Here's how the part is built. I have some questions about the finished solid (model axes, mm). A direction names the side the tool comes from. Give positions to 0.01 mm unless a question says otherwise; leave off trailing zeros. Loops run counter-clockwise (first coordinate to the right, second up) from the corner with the lowest first, then second, coordinate; pieces in that order, holes last. Notation, with made-up numbers: (-26, -10) - (-11, -10) arc R30 ccw to (-11, 15) - close; hole circle Ø6 at (-24, -5). An arc over 180 degrees is marked (long way). Use a Markdown table: item, result.
from build123d import *

# Parameters (mm, degrees)
SM_BASE_FLANGE_1_DEPTH = 2.5
HOLE_WIZARD_M41_D      = 3.3
OTHER_START            = 45.056896686
OTHER_7_OUTLINE_R      = 1.65
OTHER_7_DEPTH          = 7.095461821
OTHER_START_2          = 22.961384977
OTHER_7_2_DEPTH        = 30
OTHER_START_3          = 31.461384977
OTHER_7_3_DEPTH        = 13
OTHER_START_4          = 39.611384977
OTHER_7_4_DEPTH        = 5.85
OTHER_START_5          = 30.461384977
OTHER_7_5_DEPTH        = 5.8499999
OTHER_7_6_DEPTH        = 8.5
OTHER_START_6          = 44.461384977
OTHER_7_7_DEPTH        = 8.5
OTHER_START_7          = 40.219785041
OTHER_7_8_DEPTH        = 2.5


with BuildPart() as part:
    # Базовая кромка1: sheet metal written as solids
    # Sketch 1 → Базовая кромка1 (new body)
    with BuildSketch(Plane.XY):
        Polygon((54.77467234, 44.461384977), (73.77467234, 44.461384977), (73.77467234, 31.461384977), (54.77467234, 31.461384977), (54.77467234, 22.961384977), (78.511603406, 22.961384977), (98.77467234, 30.461384977), (98.77467234, 45.461384977), (78.77467234, 52.961384977), (54.77467234, 52.961384977), align=None)
    extrude(amount=-SM_BASE_FLANGE_1_DEPTH)

    # Отверстие обработанное метчиком M41 (through all)
    with Locations(Plane.XY):
        with Locations((83.77467234, 37.961384977), (95.77467234, 37.961384977)):
            Hole(HOLE_WIZARD_M41_D / 2)

    # Other 7: read off the stored shape, not the designer's step
    # Other 7 outline → Other 7 (cut)
    with BuildSketch(Plane(origin=(0, 0, 0), x_dir=(0.819152044288991, 0, -0.5735764363510472), z_dir=(0.5735764363510472, 0, 0.8191520442889911)).offset(OTHER_START)):
        with Locations((72.715175855, 37.961384977)):
            Circle(OTHER_7_OUTLINE_R)
    extrude(amount=OTHER_7_DEPTH, mode=Mode.SUBTRACT)

    # Other 7 2 outline → Other 7 2 (cut)
    with BuildSketch(Plane(origin=(0, 0, 0), x_dir=(1, 0, 0), z_dir=(0, 1, 0)).offset(OTHER_START_2)):
        with BuildLine():
            Line((98.77467234, 2.5), (78.050042356, 2.5))
            Line((78.050042356, 2.5), (75.641921753, 0.813815801))
            ThreePointArc((75.641921753, 0.813815801), (74.414003887, 0.208273722), (73.06082779, 0))
            Line((73.06082779, 0), (98.77467234, 0))
            Line((98.77467234, 0), (98.77467234, 2.5))
        make_face()
    extrude(amount=OTHER_7_2_DEPTH, mode=Mode.SUBTRACT)

    # Other 7 3 outline → Other 7 3 (cut)
    with BuildSketch(Plane(origin=(0, 0, 0), x_dir=(1, 0, 0), z_dir=(0, 1, 0)).offset(OTHER_START_3)):
        with BuildLine():
            Line((75.641921753, 0.813815801), (75.876326575, 0.977947824))
            Line((75.876326575, 0.977947824), (74.810574168, 2.5))
            Line((74.810574168, 2.5), (73.77467234, 2.5))
            Line((73.77467234, 2.5), (73.77467234, 0.056980086))
            ThreePointArc((73.77467234, 0.056980086), (74.751199059, 0.329550987), (75.641921753, 0.813815801))
        make_face()
    extrude(amount=OTHER_7_3_DEPTH, mode=Mode.SUBTRACT)

    # Other 7 4 outline → Other 7 4 (add)
    with BuildSketch(Plane(origin=(0, 0, 0), x_dir=(1, 0, 0), z_dir=(0, 1, 0)).offset(OTHER_START_4)):
        Polygon((78.050042356, 2.5), (96.355127682, 15.317358733), (94.921186591, 17.365238843), (74.442385484, 3.025827935), (74.810574168, 2.5), align=None)
    extrude(amount=OTHER_7_4_DEPTH)

    # Other 7 5 outline → Other 7 5 (add)
    with BuildSketch(Plane(origin=(0, 0, 0), x_dir=(1, 0, 0), z_dir=(0, 1, 0)).offset(OTHER_START_5)):
        Polygon((78.050042356, 2.5), (96.355127682, 15.317358733), (94.921186591, 17.365238843), (74.442385484, 3.025827935), (74.810574168, 2.5), align=None)
    extrude(amount=OTHER_7_5_DEPTH)

    # Other 7 6 outline → Other 7 6 (add)
    with BuildSketch(Plane(origin=(0, 0, 0), x_dir=(1, 0, 0), z_dir=(0, 1, 0)).offset(OTHER_START_2)):
        with BuildLine():
            Line((74.810574168, 2.5), (74.442385484, 3.025827935))
            Line((74.442385484, 3.025827935), (74.207980662, 2.861695911))
            ThreePointArc((74.207980662, 2.861695911), (73.662239388, 2.592566099), (73.06082779, 2.5))
            Line((73.06082779, 2.5), (74.810574168, 2.5))
        make_face()
    extrude(amount=OTHER_7_6_DEPTH)

    # Other 7 7 outline → Other 7 7 (add)
    with BuildSketch(Plane(origin=(0, 0, 0), x_dir=(1, 0, 0), z_dir=(0, 1, 0)).offset(OTHER_START_6)):
        with BuildLine():
            Line((74.810574168, 2.5), (74.442385484, 3.025827935))
            Line((74.442385484, 3.025827935), (74.207980662, 2.861695911))
            ThreePointArc((74.207980662, 2.861695911), (73.662239388, 2.592566099), (73.06082779, 2.5))
            Line((73.06082779, 2.5), (74.810574168, 2.5))
        make_face()
    extrude(amount=OTHER_7_7_DEPTH)

    # Other 7 8 outline → Other 7 8 (add)
    with BuildSketch(Plane(origin=(0, 0, 0), x_dir=(0.819152044288991, 0, -0.5735764363510472), z_dir=(0.5735764363510472, 0, 0.8191520442889911)).offset(OTHER_START_7)):
        Polygon((87.715175855, 45.461384977), (67.715175855, 52.961384977), (62.715175855, 52.961384977), (62.715175855, 45.461384977), align=None)
        Polygon((67.452106922, 22.961384977), (87.715175855, 30.461384977), (62.715175855, 30.461384977), (62.715175855, 22.961384977), align=None)
        with BuildLine():
            Line((87.715175855, 36.311384877), (87.715175855, 39.611384977))
            Line((87.715175855, 39.611384977), (84.715175855, 39.611384977))
            ThreePointArc((84.715175855, 39.611384977), (86.365175855, 37.961384977), (84.715175855, 36.311384977))
            Line((84.715175855, 36.311384977), (87.715175855, 36.311384877))
        make_face()
        with BuildLine():
            ThreePointArc((84.715175855, 36.311384977), (83.065175855, 37.961384977), (84.715175855, 39.611384977))
            Line((84.715175855, 39.611384977), (72.715175855, 39.611384977))
            ThreePointArc((72.715175855, 39.611384977), (74.365175855, 37.961384977), (72.715175855, 36.311384977))
            Line((72.715175855, 36.311384977), (84.715175855, 36.311384977))
        make_face()
        with BuildLine():
            ThreePointArc((72.715175855, 36.311384977), (71.065175855, 37.961384977), (72.715175855, 39.611384977))
            Line((72.715175855, 39.611384977), (62.715175855, 39.611384977))
            Line((62.715175855, 39.611384977), (62.715175855, 36.311384877))
            Line((62.715175855, 36.311384877), (72.715175855, 36.311384977))
        make_face()
    extrude(amount=OTHER_7_8_DEPTH)


solid = part.part
(1) Suppose I cut it at A-A on x = 63.5. Write out the boundary of the cut face in (y, z).
A:
| item | result |
|---|---|
| outline | (22.96, -2.5) - (31.46, -2.5) - (31.46, 0) - (22.96, 0) - close; (44.46, -2.5) - (52.96, -2.5) - (52.96, 0) - (44.46, 0) - close |
(2) We'd pull the mould along Y, two halves only. Please class faces 3 (the face through (64, 27, 0)), 4 (the face through (65, 31.461, -1)), 5 (the face through (65, 44.461, -1)), 6 (the face through (67, 22.961, -2)): pulls with the +Y half, pulls with the -Y half, needs draft (parallel to the pull), parting line crosses it, or undercut.
A:
| item | result |
|---|---|
| face 3 | needs draft |
| face 4 | undercut |
| face 5 | undercut |
| face 6 | pulls with the -Y half |
(3) Suppose I cut it at B-B on y = 41.75. Write out the boundary of the cut face in (x, z), plus the area to 3 significant figures.
A:
| item | result |
|---|---|
| outline | (74.44, -3.03) - (94.92, -17.37) - (96.36, -15.32) - (75.88, -0.98) - close |
| area | 62.5 mm2 |
(4) Will these pins go through, and if not, where does the flat tip stop? pin 1 (4 mm diameter, centred on y = 34.5, z = -8, fed in from +X); pin 2 (4 mm diameter, centred on x = 60, y = 47, fed in from -Z); pin 3 (10 mm diameter, centred on y = 44, z = -6.5, fed in from +X).
A:
| item | result |
|---|---|
| pin 1 | x = 88.76 |
| pin 2 | z = -2.5 |
| pin 3 | x = 90.9 |
(5) If I drill on line 1 (Z direction, x = 68, y = 26.5); line 2 (Y direction, x = 61, z = -1.25); line 3 (X direction, y = 39.75, z = -14), over which ranges is the centre line in solid material (lowest first)?
A:
| item | result |
|---|---|
| line 1 | -2.5 to 0 |
| line 2 | 22.96 to 31.46, 44.46 to 52.96 |
| line 3 | 90.12 to 94.47 |
(6) Suppose I cut it at D-D on x = 90.5. Write out the boundary of the cut face in (y, z), plus the area to 3 significant figures.
A:
| item | result |
|---|---|
| outline | (27.82, -11.22) - (28.46, -14.27) - (47.49, -14.27) - (48.14, -11.22) - close |
| area | 60.0 mm2 |
(7) On a 3-axis mill with a long thin cutter (end or side, diameter ignored), from which of +Z, -Z, +X, -X, +Y, -Y can I reach the whole of each face in a straight line? I mean faces 1 (the face through (64, 49, -2.5)), 2 (the face through (68, 52.961, -2)). Say none if no direction works.
A:
| item | result |
|---|---|
| face 1 | -Z, -X, +Y, -Y |
| face 2 | +Z, -Z, +X, -X, +Y |
(8) Suppose I cut it at C-C on z = -10.25. Write out the boundary of the cut face in (x, y), plus the area to 3 significant figures.
A:
| item | result |
|---|---|
| outline | (84.76, 25.87) - (89.12, 27.19) - (89.12, 48.77) - (84.76, 50.11) - close |
| area | 99.9 mm2 |
